Geometry check sheet. Reference: the model listing, model coordinates, mm. Coordinates: 2 decimals unless noted, no trailing zeros. Write each loop counter-clockwise with the first axis right and the second up, starting at its lowest first coordinate (ties: lowest second). Pieces come first, ordered by that corner, then holes. Notation, with made-up numbers: (27.25, 33) -> (44.25, 33) arc R18 cw to (44.25, 40) -> close; hole circle Ø1 at (-14, 27). An arc over 180 degrees is marked (long way). Answer in a Markdown table with one row per item. Add a question column.
1. Depth check by flat-ended pin: P1, Ø3, axis at x = -26.5, y = 5, coming from the +Z side; P2, Ø5, axis at x = -104.5, y = 6, coming from the -Z side; P3, Ø5, axis at x = 105, y = 3.5, coming from the -Z side. Enter the tip coordinate at first touch or a pass-through.
2. Cross-section at C-C on z = 52.5. Record the cut outline in (x, y) (3 decimals).
3. Scan lines: L1, parallel to Z at x = 38.5, y = 4 (3 decimals); L2, parallel to X at y = 4.75, z = 20; L3, parallel to X at y = 4.75, z = 19.5. Record each from-to range of solid material in increasing order. Write a range as from..to.
4. Cross-section at B-B on z = 37.5. Record the cut outline in (x, y) (3 decimals), and give its area (3 significant figures).
5. Cross-section at D-D on y = 6. Record the cut outline in (x, z) (3 decimals), and give its area (3 significant figures).
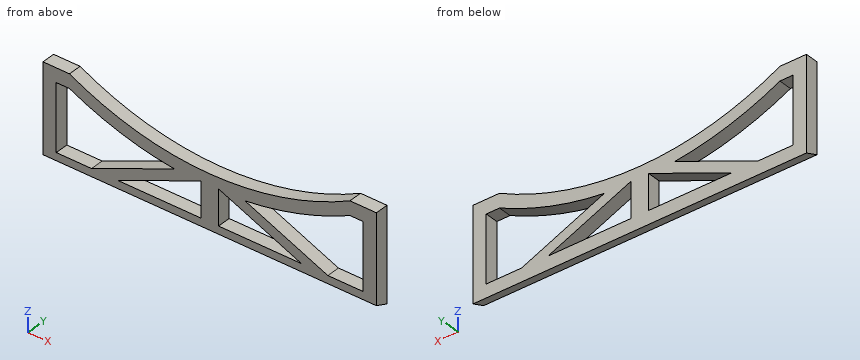
```python
from build123d import *

# Parameters (mm, degrees)
BOSS_EXTRUDE1_DEPTH = 9.525
CHAMFER1_SIZE2      = 3.93484735
CHAMFER1_SIZE       = 9.525
CUT_EXTRUDE1_DEPTH  = 138.853926046


with BuildPart() as part:
    # Sketch1 → Boss-Extrude1 (new body)
    with BuildSketch(Plane(origin=(0, 0, 0), x_dir=(1, 0, 0), z_dir=(0, 1, 0))):
        with BuildLine():
            Line((-119.85625, 0), (119.85625, 0))
            Line((119.85625, 0), (119.85625, -67.43484735))
            Line((119.85625, -67.43484735), (100.80625, -67.43484735))
            ThreePointArc((100.80625, -67.43484735), (0, -42.456061365), (-100.80625, -67.43484735))
            Line((-100.80625, -67.43484735), (-119.85625, -67.43484735))
            Line((-119.85625, -67.43484735), (-119.85625, 0))
        make_face()
    extrude(amount=BOSS_EXTRUDE1_DEPTH)

    # Chamfer1
    chamfer1_edges = [part.edges().sort_by_distance(p)[0] for p in [
        (0, 0, 0),
    ]]
    chamfer1_side = [part.faces().sort_by_distance(p)[0] for p in [
        (0, 0.078696947, 0),
    ]]
    chamfer(chamfer1_edges, length=CHAMFER1_SIZE - 0.0001, length2=CHAMFER1_SIZE2 - 0.0001, reference=chamfer1_side[0])  # a hair under: the kernel refuses the full size

    # Sketch3 → Cut-Extrude1 (cut, through all)
    with BuildSketch(Plane(origin=(0, 9.525, 0), x_dir=(1, 0, 0), z_dir=(0, 1, 0))):
        with BuildLine():
            Line((-110.33125, -57.346859726), (-110.33125, -9.525))
            Line((-110.33125, -9.525), (-84.93125, -9.525))
            Line((-84.93125, -9.525), (-25.4, -34.925))
            ThreePointArc((-25.4, -34.925), (-64.091257853, -42.812771399), (-100.80625, -57.346859726))
            Line((-100.80625, -57.346859726), (-110.33125, -57.346859726))
        make_face()
        Polygon((-65.88125, -9.525), (-6.35, -34.925), (-6.35, -9.525), align=None)
        with BuildLine():
            Line((110.33125, -57.346859726), (100.80625, -57.346859726))
            ThreePointArc((100.80625, -57.346859726), (64.091257853, -42.812771399), (25.4, -34.925))
            Line((25.4, -34.925), (84.93125, -9.525))
            Line((84.93125, -9.525), (110.33125, -9.525))
            Line((110.33125, -9.525), (110.33125, -57.346859726))
        make_face()
        Polygon((6.35, -9.525), (65.88125, -9.525), (6.35, -34.925), align=None)
    extrude(amount=-CUT_EXTRUDE1_DEPTH, mode=Mode.SUBTRACT)


solid = part.part
```
Results found:
| question | item | result |
|---|---|---|
| 1 | P1 | stops at z = 44.28 |
| 1 | P2 | stops at z = 0.42 |
| 1 | P3 | stops at z = 1.46 |
| 2 | outline | (-119.856, 0) -> (-110.331, 0) -> (-110.331, 9.525) -> (-119.856, 9.525) -> close; (-90.498, 0) -> (-65.085, 0) -> (-65.085, 9.525) -> (-90.498, 9.525) -> close; (65.085, 0) -> (90.498, 0) -> (90.498, 9.525) -> (65.085, 9.525) -> close; (110.331, 0) -> (119.856, 0) -> (119.856, 9.525) -> (110.331, 9.525) -> close |
| 3 | L1 | z = 2.282..9.525, 21.208..29.336, 36.806..45.917 |
| 3 | L2 | x = -119.86..-110.33, -60.38..-41.33, -6.35..6.35, 41.33..60.38, 110.33..119.86 |
| 3 | L3 | x = -119.86..-110.33, -61.55..-42.5, -6.35..6.35, 42.5..61.55, 110.33..119.86 |
| 4 | outline | (-119.856, 0) -> (-110.331, 0) -> (-110.331, 9.525) -> (-119.856, 9.525) -> close; (-42.299, 0) -> (42.299, 0) -> (42.299, 9.525) -> (-42.299, 9.525) -> close; (110.331, 0) -> (119.856, 0) -> (119.856, 9.525) -> (110.331, 9.525) -> close |
| 4 | area | 987 mm^2 |
| 5 | outline | (-119.856, 1.456) -> (119.856, 1.456) -> (119.856, 67.435) -> (100.806, 67.435) arc R215.9 cw to (-100.806, 67.435) -> (-119.856, 67.435) -> close; hole (-110.331, 9.525) -> (-84.931, 9.525) -> (-25.4, 34.925) arc R224.87 cw to (-100.806, 57.347) -> (-110.331, 57.347) -> close; hole (-65.881, 9.525) -> (-6.35, 9.525) -> (-6.35, 34.925) -> close; hole (6.35, 9.525) -> (65.881, 9.525) -> (6.35, 34.925) -> close; hole (25.4, 34.925) -> (84.931, 9.525) -> (110.331, 9.525) -> (110.331, 57.347) -> (100.806, 57.347) arc R224.87 cw to start |
| 5 | area | 6,350 mm^2 |
